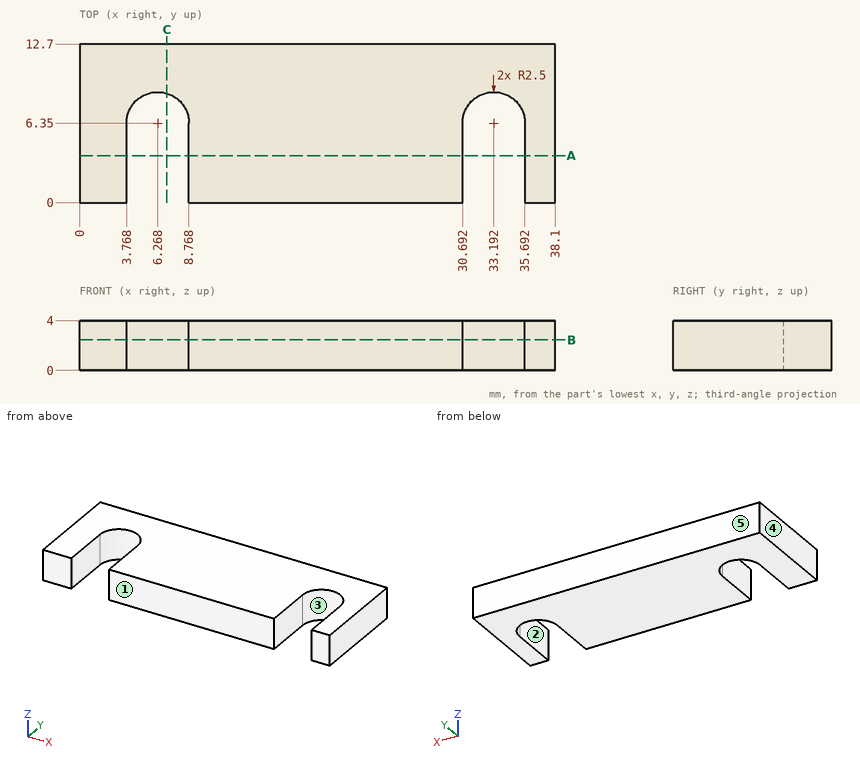
Verification items for this drawing (mm, ordinates from the low corner). A direction names the side the tool comes from. Coordinates: 2 decimals unless noted, no trailing zeros. Loops run counter-clockwise (first coordinate to the right, second up) from the corner with the lowest first, then second, coordinate; pieces in that order, holes last. Notation, with made-up numbers: (76, 54.5) - (134, 54.5) arc R24 cw to (134, 79.5) - close; hole circle Ø11 at (-20, 74). An arc over 180 degrees is marked (long way). One line per item, written item: value. Start each with the question number.
(1) Mould release check, pull along X, two halves, no side actions. Record for the marked faces 3, 4 and 5: released by +X, released by -X, zero draft, split by the parting line, or undercut.
(2) Cross-section at C-C on x = 7. Enter the section's corners in (y, z), plus the area to 3 significant figures.
(3) Cross-section at A-A on y = 3.75. Enter the section's corners in (x, z), plus the area to 3 significant figures.
(4) Material ranges on line 1 (X direction, y = 2.25, z = 2.9); line 2 (X direction, y = 7, z = 0.5); line 3 (Y direction, x = 34, z = 2.6), recorded low to high. Write a range as [from, to].
(5) Cross-section at B-B on z = 2.45. Enter the section's corners in (x, y), plus the area to 3 significant figures.
(6) Tool access check on the marked faces 1 and 2. Record the directions out of +Z, -Z, +X, -X, +Y, -Y that give a thin tool (end or side, any length) a straight path to the whole face; none if there is none.
Results below:
1. face 3: undercut
1. face 4: released by -X
1. face 5: zero draft
2. outline: (8.74, 0) - (12.7, 0) - (12.7, 4) - (8.74, 4) - close
2. area: 15.8 mm2
3. outline: (0, 0) - (3.77, 0) - (3.77, 4) - (0, 4) - close; (8.77, 0) - (30.69, 0) - (30.69, 4) - (8.77, 4) - close; (35.69, 0) - (38.1, 0) - (38.1, 4) - (35.69, 4) - close
3. area: 112 mm2
4. line 1: x = [0, 3.77], [8.77, 30.69], [35.69, 38.1]
4. line 2: x = [0, 3.85], [8.68, 30.78], [35.61, 38.1]
4. line 3: y = [8.72, 12.7]
5. outline: (0, 0) - (3.77, 0) - (3.77, 6.35) arc R2.5 cw to (8.77, 6.35) - (8.77, 0) - (30.69, 0) - (30.69, 6.35) arc R2.5 cw to (35.69, 6.35) - (35.69, 0) - (38.1, 0) - (38.1, 12.7) - (0, 12.7) - close
5. area: 401 mm2
6. face 1: +Z, -Z, +X, -X, -Y
6. face 2: +Z, -Z, -Y
